Autodesk Inventor part; units mm, degrees
ref_plane "YZ Plane" through (0, 0, 0) normal (1, 0, 0) x (0, 1, 0)
ref_plane "XZ Plane" through (0, 0, 0) normal (0, 1, 0) x (-1, 0, 0)
ref_plane "XY Plane" through (0, 0, 0) normal (0, 0, 1) x (1, 0, 0)
sketch "Sketch1" plane through (0, 0, 0) normal (0, 1, 0) x (-1, 0, 0)
  line L0 (10.9985, 0) -> (5.4993, -9.525)
  line L1 (5.4993, -9.525) -> (-5.4993, -9.525)
  line L2 (-5.4993, -9.525) -> (-10.9985, 0)
  line L3 (-10.9985, 0) -> (-5.4993, 9.525)
  line L4 (-5.4993, 9.525) -> (5.4993, 9.525)
  line L5 (5.4993, 9.525) -> (10.9985, 0)
  point P0 (0, 0)
  point P1 (0, 0)
  dimension "d0" = 9.525
extrude "Extrusion1" add sketch "Sketch1" along normal blind 6.35
sketch "Sketch2" plane through (0, 6.35, 0) normal (0, 1, 0) x (1, 0, 0)
  circle A0 centre (0, 0) radius 4.7625
  dimension "d3" = 9.525
extrude "Extrusion2" add sketch "Sketch2" along normal blind 63.5
sketch "Sketch3" plane through (0, 0, 0) normal (0, -1, 0) x (1, 0, 0)
  point P0 (0, 0)
  point P1 (0, 0)
properties part number "3-8 2.5 Inch Hex Bolt"
The listing builds one solid part. Answer for the finished solid, in the listing's coordinates (mm). A direction names the side the tool comes from. Give positions to 0.01 mm unless a question says otherwise; leave off trailing zeros. Order: outer loops, then holes, each group sorted by start corner. A loop starts at its lowest first (then second) coordinate and runs counter-clockwise, first axis right, second up. Notation, with made-up numbers: (35, 88) - (45, 88) arc R31 ccw to (45, 117) - close; hole circle Ø1 at (-29, -36.75). An arc over 180 degrees is marked (long way). Answer as CSV lines item,"result".
Q1. Each of these flat-tipped pins is pushed along its axis until it touches: pin 1 Ø1 at (y, z) = (47.5, 1.5) entering from -X; pin 2 Ø3 at (x, y) = (8, 53) entering from -Z; pin 3 Ø8 at (x, y) = (-5.5, 29) entering from -Z; pin 4 Ø1 at (x, y) = (-1, 60.5) entering from -Z. Where does it stop, or does it pass through?
Answer key:
pin 1,"stops at x = -4.66"
pin 2,"passes through"
pin 3,"stops at z = -4.52"
pin 4,"stops at z = -4.74"
Q2. A cutting plane is placed at C-C, the plane z = -3. Determine the outline of the cut face in (x, y), and give its area (3 significant figures).
Answer key:
outline,"(-9.27, 0) - (9.27, 0) - (9.27, 6.35) - (3.7, 6.35) - (3.7, 69.85) - (-3.7, 69.85) - (-3.7, 6.35) - (-9.27, 6.35) - close"
area,"587 mm^2"
Q3. Which of the six approach directions +Z, -Z, +X, -X, +Y, -Y give full straight-line access (tool end or side, diameter ignored) to faces 1 (the face through (0, 3, 9.525)), 2 (the face through (-3.78, 37.66, -2.9))?
Answer key:
face 1,"+Z, +X, -X, +Y, -Y"
face 2,"+Y"
Q4. A cutting plane is placed at B-B, the plane y = 65. Determine the outline of the cut face in (x, z) (1 decimal), and give its area (3 significant figures).
Answer key:
outline,"circle Ø9.5 at (0, 0)"
area,"71.3 mm^2"
Q5. A cutting plane is placed at D-D, the plane x = -6.75. Determine the outline of the cut face in (y, z), and give its area (3 significant figures).
Answer key:
outline,"(0, -7.36) - (6.35, -7.36) - (6.35, 7.36) - (0, 7.36) - close"
area,"93.5 mm^2"
Q6. Straight lines are drawn through the part: L1, parallel to Y at x = 3.75, z = -4; L2, parallel to Z at x = 0.25, y = 58.5. For each, find the intervals that lie inside material, in ascending order.
Answer key:
L1,"y = 0 to 6.35"
L2,"z = -4.76 to 4.76"
